from build123d import *

# Parameters (mm, degrees)
SKETCH1_W                      = 40
SKETCH1_H                      = 700
BASE_FLANGE1_DEPTH             = 3.2
EDGE_FLANGE1_STRIP_W           = 16.8
EDGE_FLANGE1_STRIP_H           = 3.2
EDGE_FLANGE1_STRIP_CUT_DEPTH   = 700
EDGE_FLANGE1_STRIP_2_W         = 16.8
EDGE_FLANGE1_STRIP_2_H         = 3.2
EDGE_FLANGE1_STRIP_CUT_2_DEPTH = 700
EDGE_FLANGE1_DEPTH             = 700
EDGE_FLANGE1_BEND_DEPTH        = 700
EDGE_FLANGE2_STRIP_W           = 16.8
EDGE_FLANGE2_STRIP_H           = 3.2
EDGE_FLANGE2_STRIP_CUT_DEPTH   = 29.6
EDGE_FLANGE2_STRIP_2_W         = 16.8
EDGE_FLANGE2_STRIP_2_H         = 3.2
EDGE_FLANGE2_STRIP_CUT_2_DEPTH = 29.6
EDGE_FLANGE2_DEPTH             = 29.6
EDGE_FLANGE2_BEND_DEPTH        = 29.6
SKETCH18_R                     = 3
CUT_EXTRUDE1_DEPTH             = 702.43940692
SKETCH29_R                     = 3
CUT_EXTRUDE12_DEPTH            = 15
CUT_EXTRUDE13_START            = -5.9
CUT_EXTRUDE13_OUTLINE_R        = 3
CUT_EXTRUDE13_DEPTH            = 3.2


# Read off the part's stored shape, not the designer's step: Cut-Extrude13
# Sheet-metal steps are written as plain solids
with BuildPart() as part:
    # Sketch1 → Base-Flange1 (new body)
    with BuildSketch(Plane.XY):
        with Locations((-0.426492134, -287.746478873)):
            Rectangle(SKETCH1_W, SKETCH1_H)
    extrude(amount=-BASE_FLANGE1_DEPTH)

    # Edge-Flange1 strip (across the edge) → Edge-Flange1 strip cut (cut)
    with BuildSketch(Plane(origin=(-20.426492134, 62.253521127, 0), x_dir=(1, 0, 0), z_dir=(0, -1, 0))):
        with Locations((-3.2, -1.6)):
            Rectangle(EDGE_FLANGE1_STRIP_W, EDGE_FLANGE1_STRIP_H)
    extrude(amount=EDGE_FLANGE1_STRIP_CUT_DEPTH, mode=Mode.SUBTRACT)

    # Edge-Flange1 strip 2 (across the edge) → Edge-Flange1 strip cut 2 (cut)
    with BuildSketch(Plane(origin=(19.573507866, -637.746478873, 0), x_dir=(-1, 0, 0), z_dir=(0, 1, 0))):
        with Locations((-3.2, -1.6)):
            Rectangle(EDGE_FLANGE1_STRIP_2_W, EDGE_FLANGE1_STRIP_2_H)
    extrude(amount=EDGE_FLANGE1_STRIP_CUT_2_DEPTH, mode=Mode.SUBTRACT)

    # Edge-Flange1 section (across the edge) → Edge-Flange1 (add)
    with BuildSketch(Plane(origin=(-20.426492134, 62.253521127, 0), x_dir=(1, 0, 0), z_dir=(0, -1, 0))):
        with BuildLine():
            Line((0, 2), (0, 16.8))
            Line((0, 16.8), (3.2, 16.8))
            Line((3.2, 16.8), (3.2, 2))
            ThreePointArc((3.2, 2), (3.785786438, 0.585786438), (5.2, 0))
            Line((5.2, 0), (5.2, -3.2))
            ThreePointArc((5.2, -3.2), (1.523044738, -1.676955262), (0, 2))
        make_face()
    extrude(amount=EDGE_FLANGE1_DEPTH)

    # Edge-Flange1 section 2 (across the edge) → Edge-Flange1 bend (add)
    with BuildSketch(Plane(origin=(19.573507866, -637.746478873, 0), x_dir=(-1, 0, 0), z_dir=(0, 1, 0))):
        with BuildLine():
            Line((0, 2), (0, 16.8))
            Line((0, 16.8), (3.2, 16.8))
            Line((3.2, 16.8), (3.2, 2))
            ThreePointArc((3.2, 2), (3.785786438, 0.585786438), (5.2, 0))
            Line((5.2, 0), (5.2, -3.2))
            ThreePointArc((5.2, -3.2), (1.523044738, -1.676955262), (0, 2))
        make_face()
    extrude(amount=EDGE_FLANGE1_BEND_DEPTH)

    # Edge-Flange2 strip (across the edge) → Edge-Flange2 strip cut (cut)
    with BuildSketch(Plane(origin=(-15.226492134, 62.253521127, -3.2), x_dir=(0, -1, 0), z_dir=(1, 0, 0))):
        with Locations((-3.2, -1.6)):
            Rectangle(EDGE_FLANGE2_STRIP_W, EDGE_FLANGE2_STRIP_H)
    extrude(amount=EDGE_FLANGE2_STRIP_CUT_DEPTH, mode=Mode.SUBTRACT)

    # Edge-Flange2 strip 2 (across the edge) → Edge-Flange2 strip cut 2 (cut)
    with BuildSketch(Plane(origin=(14.373507866, -637.746478873, -3.2), x_dir=(0, 1, 0), z_dir=(-1, 0, 0))):
        with Locations((-3.2, -1.6)):
            Rectangle(EDGE_FLANGE2_STRIP_2_W, EDGE_FLANGE2_STRIP_2_H)
    extrude(amount=EDGE_FLANGE2_STRIP_CUT_2_DEPTH, mode=Mode.SUBTRACT)

    # Edge-Flange2 section (across the edge) → Edge-Flange2 (add)
    with BuildSketch(Plane(origin=(-15.226492134, 62.253521127, -3.2), x_dir=(0, -1, 0), z_dir=(1, 0, 0))):
        with BuildLine():
            Line((0, 2), (0, 36.8))
            Line((0, 36.8), (3.2, 36.8))
            Line((3.2, 36.8), (3.2, 2))
            ThreePointArc((3.2, 2), (3.785786438, 0.585786438), (5.2, 0))
            Line((5.2, 0), (5.2, -3.2))
            ThreePointArc((5.2, -3.2), (1.523044738, -1.676955262), (0, 2))
        make_face()
    extrude(amount=EDGE_FLANGE2_DEPTH)

    # Edge-Flange2 section 2 (across the edge) → Edge-Flange2 bend (add)
    with BuildSketch(Plane(origin=(14.373507866, -637.746478873, -3.2), x_dir=(0, 1, 0), z_dir=(-1, 0, 0))):
        with BuildLine():
            Line((0, 2), (0, 36.8))
            Line((0, 36.8), (3.2, 36.8))
            Line((3.2, 36.8), (3.2, 2))
            ThreePointArc((3.2, 2), (3.785786438, 0.585786438), (5.2, 0))
            Line((5.2, 0), (5.2, -3.2))
            ThreePointArc((5.2, -3.2), (1.523044738, -1.676955262), (0, 2))
        make_face()
    extrude(amount=EDGE_FLANGE2_BEND_DEPTH)

    # Sketch18 → Cut-Extrude1 (cut, through all)
    with BuildSketch(Plane(origin=(0, 62.253521127, 0), x_dir=(1, 0, 0), z_dir=(0, 1, 0))):
        with Locations(Location((0, 22.6, 0), (0, 0, 270))):
            Circle(SKETCH18_R)
    extrude(amount=-CUT_EXTRUDE1_DEPTH, mode=Mode.SUBTRACT)

    # Sketch29 → Cut-Extrude12 (cut)
    with BuildSketch(Plane(origin=(98.729905779, -312.144507489, -5.9), x_dir=(-1, 0, 0), z_dir=(0, 0, -1))):
        with Locations((100.456397914, 211.698028616)):
            Circle(SKETCH29_R)
        with Locations((100.456397914, 171.698028616)):
            Circle(SKETCH29_R)
        with Locations((100.456397914, 111.698028616)):
            Circle(SKETCH29_R)
        with Locations((100.456397914, 51.698028616)):
            Circle(SKETCH29_R)
        with Locations((100.456397914, -8.301971384)):
            Circle(SKETCH29_R)
        with Locations((100.456397914, -68.301971384)):
            Circle(SKETCH29_R)
        with Locations((100.456397914, -128.301971384)):
            Circle(SKETCH29_R)
        with Locations((100.456397914, -188.301971384)):
            Circle(SKETCH29_R)
        with Locations((100.456397914, -248.301971384)):
            Circle(SKETCH29_R)
    extrude(amount=-CUT_EXTRUDE12_DEPTH, mode=Mode.SUBTRACT)

    # Cut-Extrude13 outline → Cut-Extrude13 (cut)
    with BuildSketch(Plane(origin=(260.729905779, -312.144507489, -5.9), x_dir=(-1, 0, 0), z_dir=(0, 0, -1)).offset(CUT_EXTRUDE13_START)):
        with BuildLine():
            ThreePointArc((262.206397914, -251.29153657), (259.456397914, -248.301971384), (262.206397914, -245.312406198))
            ThreePointArc((262.206397914, -245.312406198), (258.956397914, -248.301971384), (262.206397914, -251.29153657))
        make_face()
        with BuildLine():
            ThreePointArc((262.206397914, 208.70846343), (259.456397914, 211.698028616), (262.206397914, 214.687593802))
            ThreePointArc((262.206397914, 214.687593802), (258.956397914, 211.698028616), (262.206397914, 208.70846343))
        make_face()
        with Locations((261.956397914, -208.301971384)):
            Circle(CUT_EXTRUDE13_OUTLINE_R)
        with Locations((261.956397914, -148.301971384)):
            Circle(CUT_EXTRUDE13_OUTLINE_R)
        with Locations((261.956397914, -88.301971384)):
            Circle(CUT_EXTRUDE13_OUTLINE_R)
        with Locations((261.956397914, -28.301971384)):
            Circle(CUT_EXTRUDE13_OUTLINE_R)
        with Locations((261.956397914, 31.698028616)):
            Circle(CUT_EXTRUDE13_OUTLINE_R)
        with Locations((261.956397914, 91.698028616)):
            Circle(CUT_EXTRUDE13_OUTLINE_R)
        with Locations((261.956397914, 151.698028616)):
            Circle(CUT_EXTRUDE13_OUTLINE_R)
    extrude(amount=CUT_EXTRUDE13_DEPTH, mode=Mode.SUBTRACT)


solid = part.part
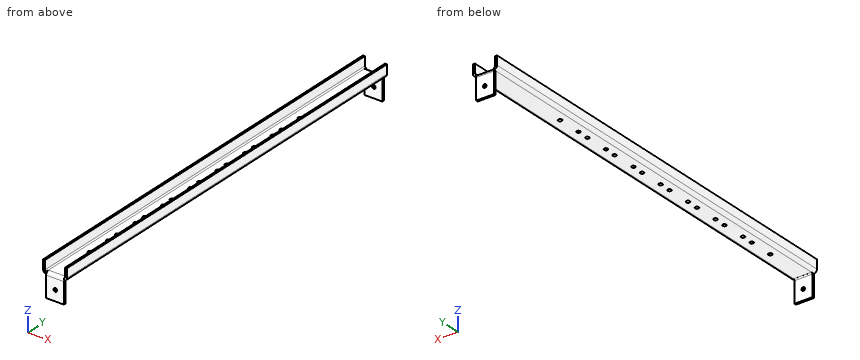
The listing builds one solid part. Answer for the finished solid, in the listing's coordinates (mm). Give positions to 0.01 mm unless a question says otherwise; leave off trailing zeros. Write each loop counter-clockwise with the first axis right and the second up, starting at its lowest first coordinate (ties: lowest second). Pieces come first, ordered by that corner, then holes.
Item 1: Flat-ended cylindrical pins translate along their axes: P1, Ø8, axis at x = -1.23, y = -280.45, coming from the -Z side; P2, Ø5, axis at x = -1.73, y = -100.45, coming from the +Z side; P3, Ø9.5, axis at x = -1.73, y = -260.45, coming from the +Z side; P4, Ø5.5, axis at y = 59.5, z = -18.5, coming from the +X side. Find the tip coordinate at first contact, or state that the pin passes through.
Item 2: Find the intervals of material crossed by line 1 along Y through (x, z) = (-14.5, -35.5); line 2 along Z through (x, y) = (7.5, -605); line 3 along Y through (x, z) = (5, -5), in increasing order.
Item 3: Section B-B, the plane y = -416.5 is taken. Write down the section's boundary in (x, z), plus the area to 3 significant figures.
Item 4: Section A-A, the plane z = -11.5 is taken. Write down the section's boundary in (x, y), plus the area to 3 significant figures.
Completed:
1. P1: stops at z = -3.2
1. P2: passes through
1. P3: stops at z = 0
1. P4: stops at x = 14.37
2. line 1: y = -637.75 to -634.55, 59.05 to 62.25
2. line 2: z = -3.2 to 0
2. line 3: y = -637.74 to -634.54, 59.04 to 62.25
3. outline: (-20.43, 2) arc R5.2 ccw to (-15.23, -3.2) - (14.37, -3.2) arc R5.2 ccw to (19.57, 2) - (19.57, 16.8) - (16.37, 16.8) - (16.37, 2) arc R2 cw to (14.37, 0) - (-15.23, 0) arc R2 cw to (-17.23, 2) - (-17.23, 16.8) - (-20.43, 16.8) - close
3. area: 226 mm2
4. outline: (-15.23, -637.75) - (14.37, -637.75) - (14.37, -634.55) - (-15.23, -634.55) - close; (-15.23, 59.05) - (14.37, 59.05) - (14.37, 62.25) - (-15.23, 62.25) - close
4. area: 189 mm2
